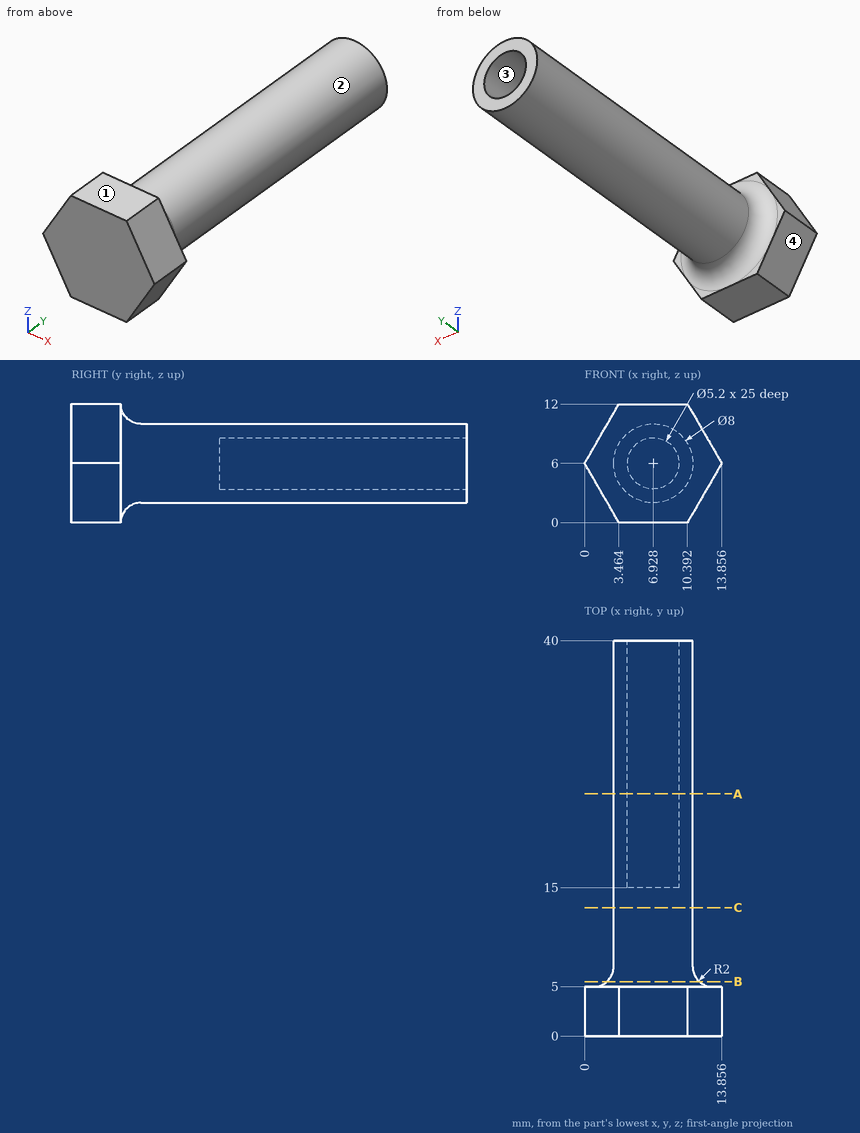
Source: three-view drawing plus pictorial views. Frame: mm from the lowest corner of the part. Give positions to 0.01 mm unless a question says otherwise; leave off trailing zeros. Write each loop counter-clockwise with the first axis right and the second up, starting at its lowest first coordinate (ties: lowest second). Pieces come first, ordered by that corner, then holes. Notation, with made-up numbers: (33, 57.25) -> (49, 57.25) arc R17 cw to (49, 61.25) -> close; hole circle Ø2 at (16, 13.25). An arc over 180 degrees is marked (long way). Answer in a Markdown table with one row per item.
(1) Ray query, line 1 along Z through (x, y) = (6.75, 37) (1 decimal); line 2 along X through (y, z) = (22, 7.25); line 3 along X through (y, z) = (8.5, 6.5). Return the intervals inside material, ascending. Write a range as [from, to].
Answers below:
| item | result |
|---|---|
| line 1 | [2, 3.4], [8.6, 10] |
| line 2 | [3.13, 4.65], [9.21, 10.73] |
| line 3 | [2.96, 10.9] |
(2) Section query A-A on y = 24.5. Return loops of the section in (x, z).
Answers below:
| item | result |
|---|---|
| outline | circle Ø8 at (6.93, 6); hole circle Ø5.2 at (6.93, 6) |
(3) Section query C-C on y = 13. Return loops of the section in (x, z).
Answers below:
| item | result |
|---|---|
| outline | circle Ø8 at (6.93, 6) |
(4) Pin query (flat end, axial travel): pin 1 (5 mm diameter, centred on x = 4, z = 3.5, fed in from -Y); pin 2 (5 mm diameter, centred on y = 32.5, z = 9.5, fed in from +X); pin 3 (6 mm diameter, centred on x = 5, y = 34.5, fed in from -Z); pin 4 (5 mm diameter, centred on x = 3, y = 11.5, fed in from +Z). Return the tip coordinate at first contact, or that it passes through.
Answers below:
| item | result |
|---|---|
| pin 1 | y = 0 |
| pin 2 | x = 10.8 |
| pin 3 | z = 2 |
| pin 4 | z = 9.74 |
(5) Section query B-B on y = 5.5. Return loops of the section in (x, z), then the cut area to 3 significant figures.
Answers below:
| item | result |
|---|---|
| outline | circle Ø9.35 at (6.93, 6) |
| area | 68.7 mm^2 |
(6) Draft query along X for the marked faces 1, 2, 3 and 4. Return one class per face: +X half, -X half, draft (parallel to the pull), parting line (faces both ways), or undercut.
Answers below:
| item | result |
|---|---|
| face 1 | draft |
| face 2 | parting line |
| face 3 | undercut |
| face 4 | -X half |
